Answer from the drawing. Dimensions are ordinates in mm from the lowest x, y and z of the part. A direction names the side the tool comes from. Round coordinates to 2 decimals unless told otherwise and drop trailing zeros. Write each loop counter-clockwise with the first axis right and the second up, starting at its lowest first coordinate (ties: lowest second). Pieces come first, ordered by that corner, then holes. Notation, with made-up numbers: (-5.75, 42.25) - (6.25, 42.25) arc R14 ccw to (6.25, 55.25) - close; hole circle Ø8 at (28, 51). An arc over 180 degrees is marked (long way). Answer as CSV lines item,"result". Start each with the question number.
1) Each of these flat-tipped pins is pushed along its axis until it touches: pin 1 (2 mm diameter, centred on x = 24.5, z = 6, fed in from -Y); pin 2 (3 mm diameter, centred on x = 7.5, z = 10, fed in from +Y); pin 3 (2 mm diameter, centred on y = 42.5, z = 5, fed in from -X); pin 4 (3 mm diameter, centred on y = 5.08, z = 7.62, fed in from -X). Where does it stop, or does it pass through?
2) Find section A-A on y = 5.08. Determine the outline of the cut face in (x, z).
3) Which of the six approach directions +Z, -Z, +X, -X, +Y, -Y give full straight-line access (tool end or side, diameter ignored) to the marked faces 1 and 2?
4) Find section B-B on x = 30. Determine the outline of the cut face in (y, z), then the cut area to 3 significant figures.
5) Consider line 1 along Z through (x, y) = (33, 5); line 2 along X through (y, z) = (2.5, 12.5); line 3 along Y through (x, z) = (16.5, 7.25). Determine where each line is inside the solid, lowest interval first.
6) Find section D-D on x = 8. Determine the outline of the cut face in (y, z).
7) For a pull along Z with two mould halves and no side action, classify the marked faces 3, 4 and 5 as +Z half, -Z half, draft (parallel to the pull), parting line (faces both ways), or undercut.
8) Find section C-C on y = 48.26. Determine the outline of the cut face in (x, z), then the cut area to 3 significant figures.
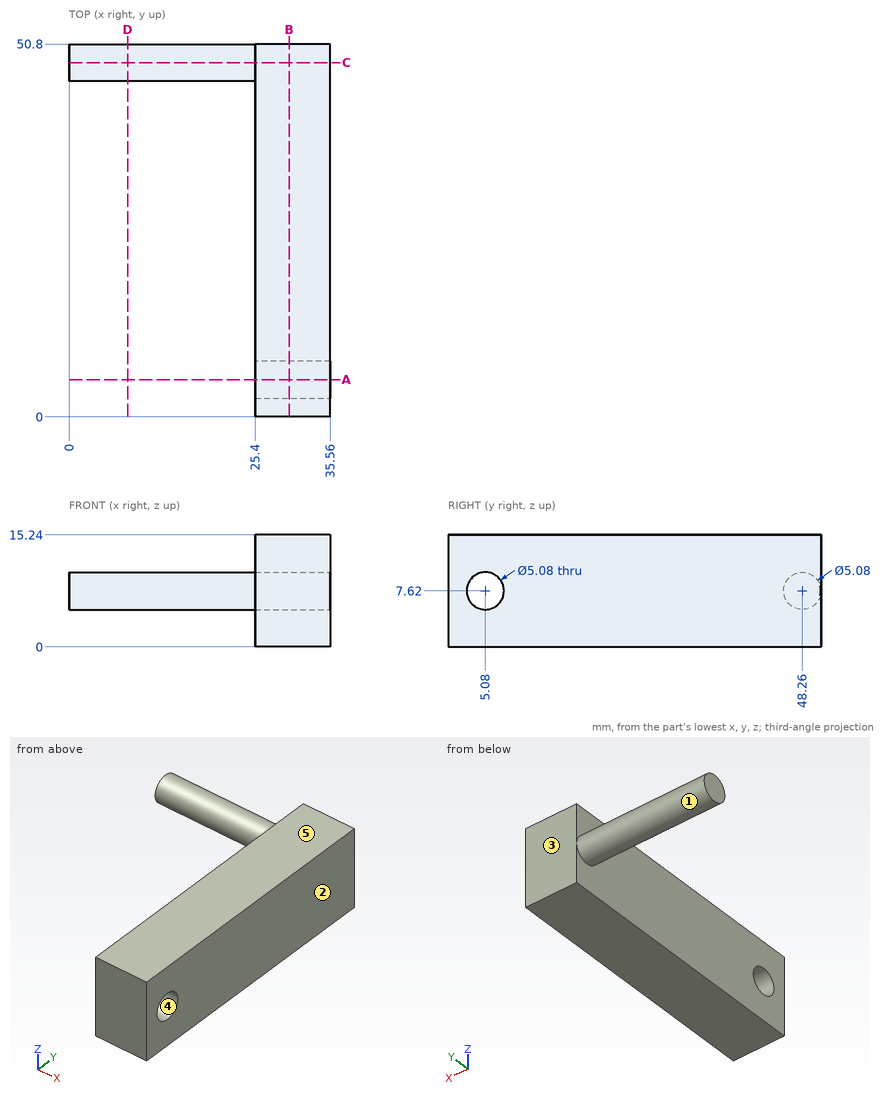
Check values:
1,pin 1,"stops at y = 0"
1,pin 2,"stops at y = 50.64"
1,pin 3,"stops at x = 25.4"
1,pin 4,"passes through"
2,outline,"(25.4, 0) - (35.56, 0) - (35.56, 5.08) - (25.4, 5.08) - close; (25.4, 10.16) - (35.56, 10.16) - (35.56, 15.24) - (25.4, 15.24) - close"
3,face 1,"-X"
3,face 2,"+Z, -Z, +X, +Y, -Y"
4,outline,"(0, 0) - (50.8, 0) - (50.8, 15.24) - (0, 15.24) - close; hole circle Ø5.08 at (5.08, 7.62)"
4,area,"754 mm^2"
5,line 1,"z = 0 to 5.08, 10.16 to 15.24"
5,line 2,"x = 25.4 to 35.56"
5,line 3,"y = 45.75 to 50.77"
6,outline,"circle Ø5.08 at (48.26, 7.62)"
7,face 3,"draft"
7,face 4,"undercut"
7,face 5,"+Z half"
8,outline,"(0, 5.08) - (25.4, 5.08) - (25.4, 0) - (35.56, 0) - (35.56, 15.24) - (25.4, 15.24) - (25.4, 10.16) - (0, 10.16) - close"
8,area,"284 mm^2"
